Part model, mm, in its own coordinate system. A direction names the side the tool comes from. Give positions to 0.01 mm unless a question says otherwise; leave off trailing zeros. Loops run counter-clockwise (first coordinate to the right, second up) from the corner with the lowest first, then second, coordinate; pieces in that order, holes last. Notation, with made-up numbers: M 25.25,-13.5 L 61.25,-13.5 A23 cw 61.25,-2.5 Z; hole C 38,45.25 d4. An arc over 180 degrees is marked long. Answer in a Markdown table with one row per item.
from build123d import *

# Parameters (mm, degrees)
SKETCH1_R                = 3.155
BOSS_EXTRUDE7_DEPTH      = 15.9
SHELL1_T                 = -2
CUT_EXTRUDE5_START       = 2
CUT_EXTRUDE5_OUTLINE_R   = 5.155
CUT_EXTRUDE5_OUTLINE_R_2 = 3.155
CUT_EXTRUDE5_DEPTH       = 11.9


# Read off the part's stored shape, not the designer's step: Cut-Extrude5
with BuildPart() as part:
    # Sketch1 → Boss-Extrude7 (new body)
    with BuildSketch(Plane(origin=(0, 0, 0), x_dir=(1, 0, 0), z_dir=(0, 1, 0))):
        with BuildLine():
            Line((-57.361665301, -13.110958237), (27.188334699, -13.110958237))
            ThreePointArc((27.188334699, -13.110958237), (41.913334699, 1.614041763), (27.188334699, 16.339041763))
            Line((27.188334699, 16.339041763), (-57.361665301, 16.339041763))
            Line((-57.361665301, 16.339041763), (-57.361665301, -13.110958237))
        make_face()
        with Locations(Location((33.498334699, 1.614041763, 0), (0, 0, 270))):
            Circle(SKETCH1_R, mode=Mode.SUBTRACT)
    extrude(amount=BOSS_EXTRUDE7_DEPTH)

    # Shell1
    shell1_openings = [part.faces().sort_by_distance(p)[0] for p in [
        (-57.361665301, 7.95, -1.614041763),
    ]]
    offset(amount=SHELL1_T, openings=shell1_openings, kind=Kind.INTERSECTION)

    # Cut-Extrude5 outline → Cut-Extrude5 (cut)
    with BuildSketch(Plane(origin=(0, 0, 0), x_dir=(1, 0, 0), z_dir=(0, 1, 0)).offset(CUT_EXTRUDE5_START)):
        with Locations((33.498334699, 1.614041763)):
            Circle(CUT_EXTRUDE5_OUTLINE_R)
        with Locations((33.498334699, 1.614041763)):
            Circle(CUT_EXTRUDE5_OUTLINE_R_2, mode=Mode.SUBTRACT)
    extrude(amount=CUT_EXTRUDE5_DEPTH, mode=Mode.SUBTRACT)


solid = part.part
(1) Saw through at C-C (y = 6). Write the cut outline in (x, z) (3 decimals), plus the area to 3 significant figures.
Recorded:
| item | result |
|---|---|
| outline | M -57.362,-16.339 L 27.188,-16.339 A14.725 ccw 27.188,13.111 L -57.362,13.111 L -57.362,11.111 L 27.188,11.111 A12.725 cw 27.188,-14.339 L -57.362,-14.339 Z |
| area | 424 mm^2 |
(2) Pin check, flat tips, straight feed: pin 1 Ø1 at (y, z) = (9, -9.5) entering from -X; pin 2 Ø2 at (y, z) = (5.5, 5) entering from -X; pin 3 Ø4 at (y, z) = (7.5, -9) entering from -X. Stop position of each tip, or through.
Recorded:
| item | result |
|---|---|
| pin 1 | stops at x = 36.76 |
| pin 2 | stops at x = 37.38 |
| pin 3 | stops at x = 35.78 |
(3) Saw through at D-D (z = 6.5). Write the cut outline in (x, y), plus the area to 3 significant figures.
Recorded:
| item | result |
|---|---|
| outline | M -57.36,0 L 39.48,0 L 39.48,15.9 L -57.36,15.9 L -57.36,13.9 L 36.99,13.9 L 36.99,2 L -57.36,2 Z |
| area | 417 mm^2 |
(4) Which spindle directions (+Z, -Z, +X, -X, +Y, -Y) get a long thin tool onto all of the face, cutting with end or side? Do faces 1 (the face through (41.91, 7.84, -1.29)), 2 (the face through (-9, 2, -2)). Say none if no direction does.
Recorded:
| item | result |
|---|---|
| face 1 | +X, +Y, -Y |
| face 2 | -X |
(5) Drill centre lines: line 1 along Z through (x, y) = (-47, 4); line 2 along Y through (x, z) = (-6, 10.75); line 3 along X through (y, z) = (9.5, -1.5). Where is each one in solid material? Low to high.
Recorded:
| item | result |
|---|---|
| line 1 | z = -16.34 to -14.34, 11.11 to 13.11 |
| line 2 | y = 0 to 2, 13.9 to 15.9 |
| line 3 | x = 39.91 to 41.91 |
(6) Saw through at B-B (z = -3.5). Write the cut outline in (x, y).
Recorded:
| item | result |
|---|---|
| outline | M -57.36,0 L 30.97,0 L 30.97,2 L -57.36,2 Z; M -57.36,13.9 L 30.97,13.9 L 30.97,15.9 L -57.36,15.9 Z; M 36.03,0 L 41.79,0 L 41.79,15.9 L 36.03,15.9 L 36.03,13.9 L 39.77,13.9 L 39.77,2 L 36.03,2 Z |
(7) Pull direction X, two halves, no side cores. Call faces 3 (the face through (39.91, 7.87, -1.33)), 4 (the face through (36.626, 14.886, -2.025)), 5 (the face through (-8, 0, -2)): +X half, -X half, draft (parallel to the pull), parting line (faces both ways), or undercut.
Recorded:
| item | result |
|---|---|
| face 3 | -X half |
| face 4 | undercut |
| face 5 | draft |
(8) Saw through at A-A (x = 15). Write the cut outline in (y, z).
Recorded:
| item | result |
|---|---|
| outline | M 0,-16.34 L 15.9,-16.34 L 15.9,13.11 L 0,13.11 Z; hole M 2,-14.34 L 13.9,-14.34 L 13.9,11.11 L 2,11.11 Z |
